Here's the drawing with two shaded views (mm, measured from the low corner). I have some questions. A direction names the side the tool comes from. Give positions to 0.01 mm unless a question says otherwise; leave off trailing zeros. Write each loop counter-clockwise with the first axis right and the second up, starting at its lowest first coordinate (ties: lowest second). Pieces come first, ordered by that corner, then holes. Notation, with made-up numbers: (-28.5, 66.25) -> (22.5, 66.25) arc R21 cw to (22.5, 92.25) -> close; hole circle Ø5 at (2, 25.5). An arc over 180 degrees is marked (long way). One line per item, written item: value.
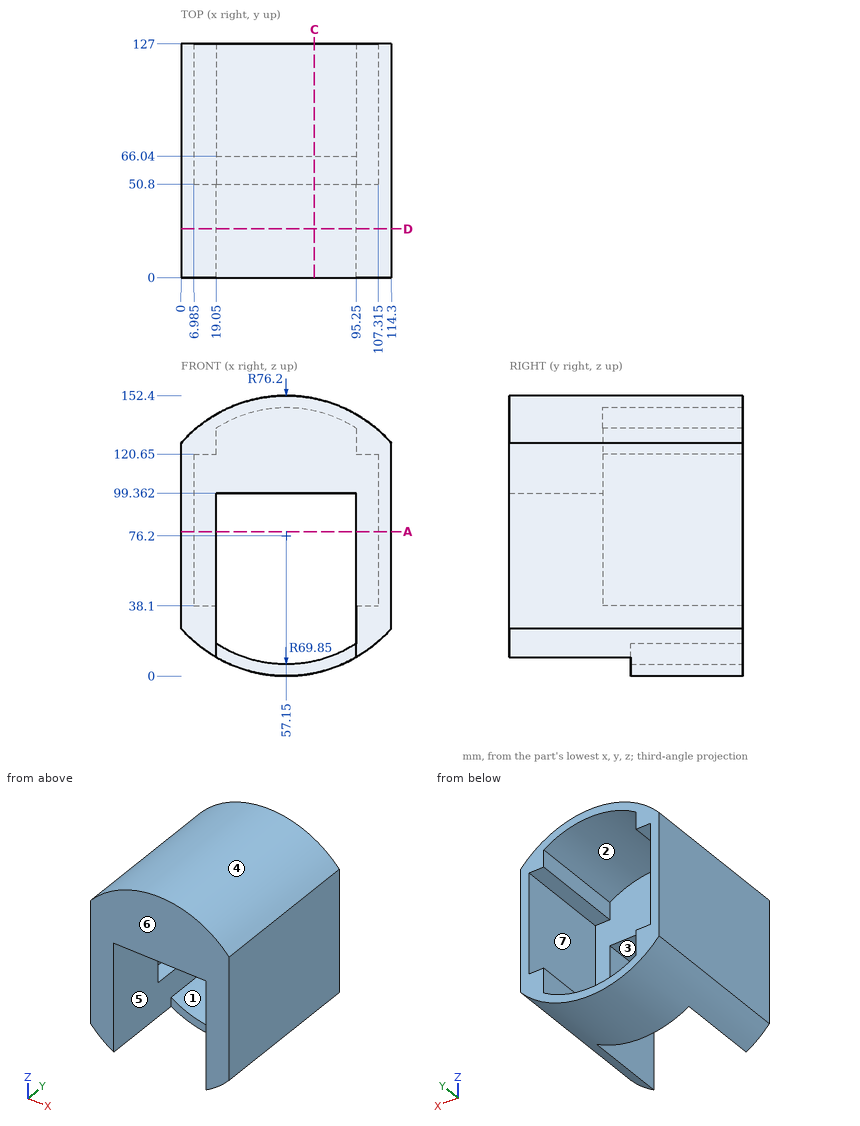
1) If we section it at A-A (z = 78.5): Write out the boundary of the cut face in (x, y) (3 decimals), and give its area (3 significant figures).
Answer list:
outline: (0, 0) -> (19.05, 0) -> (19.05, 50.8) -> (6.985, 50.8) -> (6.985, 127) -> (0, 127) -> close; (95.25, 0) -> (114.3, 0) -> (114.3, 127) -> (107.315, 127) -> (107.315, 50.8) -> (95.25, 50.8) -> close
area: 3,000 mm^2
2) If we section it at C-C (x = 72.5): Write out the boundary of the cut face in (y, z).
Answer list:
outline: (0, 99.36) -> (50.8, 99.36) -> (50.8, 144.34) -> (127, 144.34) -> (127, 150.84) -> (0, 150.84) -> close; (66.04, 1.56) -> (127, 1.56) -> (127, 8.06) -> (66.04, 8.06) -> close
3) We'd pull the mould along X, two halves only. Please class the marked faces 4, 5, 6 and 7: released by +X, released by -X, zero draft, split by the parting line, or undercut.
Answer list:
face 4: split by the parting line
face 5: undercut
face 6: zero draft
face 7: undercut
4) Will these pins go through, and if not, where does the flat tip stop? pin 1 (5.5 mm diameter, centred on x = 51, z = 7.5, fed in from -Y); pin 2 (1 mm diameter, centred on x = 82, y = 20.5, fed in from -Z); pin 3 (3.5 mm diameter, centred on x = 98.5, y = 89, fed in from +Z).
Answer list:
pin 1: stops at y = 66.04
pin 2: stops at z = 99.36
pin 3: stops at z = 141.3
5) For the marked faces 1, 2 and 3, which set-ups out of +Z, -Z, +X, -X, +Y, -Y let a thin tool reach every point of the face, with its end or its side?
Answer list:
face 1: +Y, -Y
face 2: +Y
face 3: -Z, +Y, -Y
6) If we section it at D-D (y = 26.5): Write out the boundary of the cut face in (x, z).
Answer list:
outline: (0, 25.8) arc R76.2 ccw to (19.05, 10.21) -> (19.05, 99.36) -> (95.25, 99.36) -> (95.25, 10.21) arc R76.2 ccw to (114.3, 25.8) -> (114.3, 126.6) arc R76.2 ccw to (0, 126.6) -> close
7) I need wall thicknesses on L1, parallel to X at y = 62, z = 75.5 (3 decimals); L2, parallel to Z at x = 59, y = 78.5; L3, parallel to Y at x = 91, z = 127.5. Which ranges of each line are inside material? Lowest first, please.
Answer list:
L1: x = 0 to 6.985, 107.315 to 114.3
L2: z = 0.02 to 6.37, 146.03 to 152.38
L3: y = 0 to 50.8
